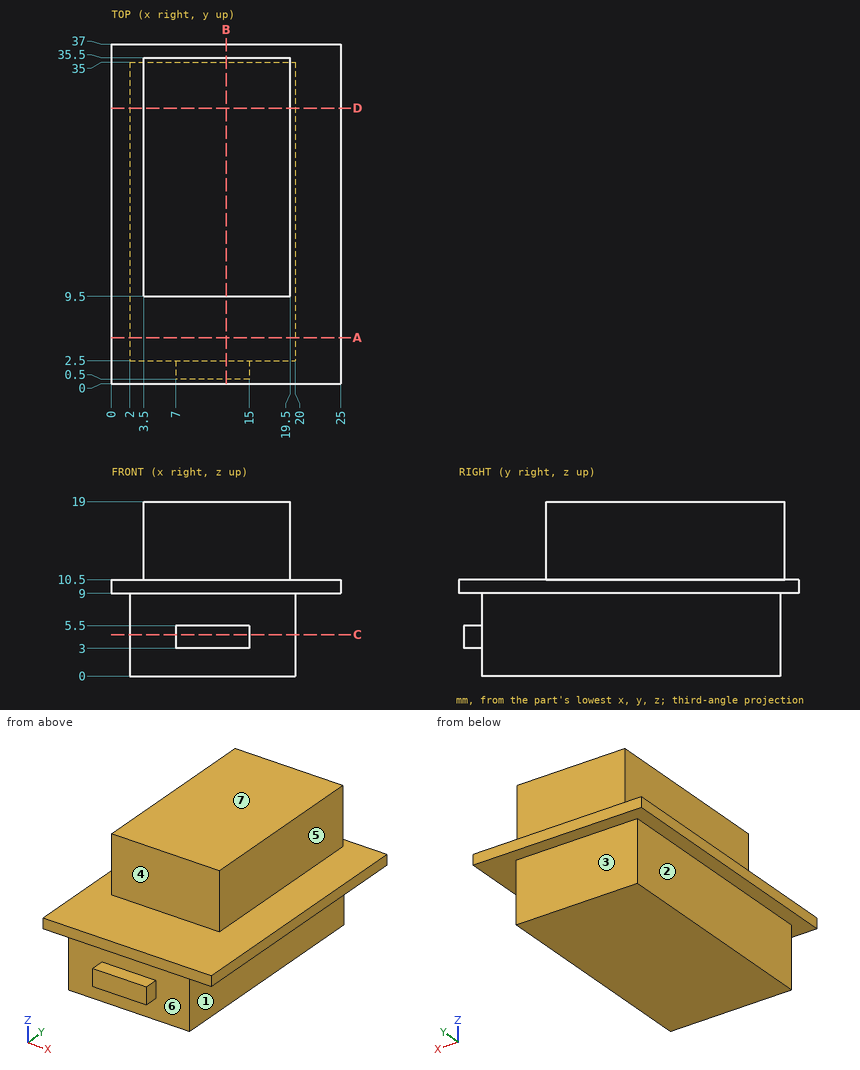
Answer from the drawing. Dimensions are ordinates in mm from the lowest x, y and z of the part. A direction names the side the tool comes from. Coordinates: 2 decimals unless noted, no trailing zeros. Loops run counter-clockwise (first coordinate to the right, second up) from the corner with the lowest first, then second, coordinate; pieces in that order, holes last. Notation, with made-up numbers: (22.5, 78) -> (38.5, 78) arc R20 cw to (38.5, 116) -> close; hole circle Ø8 at (25, -5). An arc over 180 degrees is marked (long way). Answer as CSV lines item,"result".
Q1. The part is cut by section C-C on z = 4.5. Write down the section's boundary in (x, y).
Findings:
outline,"(2, 2.5) -> (7, 2.5) -> (7, 0.5) -> (15, 0.5) -> (15, 2.5) -> (20, 2.5) -> (20, 35) -> (2, 35) -> close"
Q2. The part is cut by section D-D on y = 30. Write down the section's boundary in (x, z).
Findings:
outline,"(0, 9) -> (2, 9) -> (2, 0) -> (20, 0) -> (20, 9) -> (25, 9) -> (25, 10.5) -> (19.5, 10.5) -> (19.5, 19) -> (3.5, 19) -> (3.5, 10.5) -> (0, 10.5) -> close"
Q3. The part is cut by section B-B on x = 12.5. Write down the section's boundary in (y, z).
Findings:
outline,"(0, 9) -> (2.5, 9) -> (2.5, 5.5) -> (0.5, 5.5) -> (0.5, 3) -> (2.5, 3) -> (2.5, 0) -> (35, 0) -> (35, 9) -> (37, 9) -> (37, 10.5) -> (35.5, 10.5) -> (35.5, 19) -> (9.5, 19) -> (9.5, 10.5) -> (0, 10.5) -> close"
Q4. For a pull along Z with two mould halves and no side action, classify the marked faces 5, 6 and 7 as +Z half, -Z half, draft (parallel to the pull), parting line (faces both ways), or undercut.
Findings:
face 5,"draft"
face 6,"undercut"
face 7,"+Z half"
Q5. The part is cut by section A-A on y = 5. Write down the section's boundary in (x, z), and give its area (4 significant figures).
Findings:
outline,"(0, 9) -> (2, 9) -> (2, 0) -> (20, 0) -> (20, 9) -> (25, 9) -> (25, 10.5) -> (0, 10.5) -> close"
area,"199.5 mm²"
Q6. Find the intervals of material crossed by probe 1 along Y at (x, z) = (11, 2.5); probe 2 along Z at (x, y) = (3.25, 24); probe 3 along X at (y, z) = (28.5, 12), in increasing order.
Findings:
probe 1,"y = 2.5 to 35"
probe 2,"z = 0 to 10.5"
probe 3,"x = 3.5 to 19.5"
Q7. Each of these flat-tipped pins is pushed along its axis until it touches: pin 1 (2.5 mm diameter, centred on y = 18.5, z = 15.5, fed in from -X); pin 2 (2 mm diameter, centred on x = 13.5, z = 5.5, fed in from -Y); pin 3 (1 mm diameter, centred on x = 12, z = 8, fed in from -Y). Where does it stop, or does it pass through?
Findings:
pin 1,"stops at x = 3.5"
pin 2,"stops at y = 0.5"
pin 3,"stops at y = 2.5"
Q8. A tool of negligible diameter and unlimited length cuts with its end or side. For the marked faces 1, 2, 3 and 4, from which of +Z, -Z, +X, -X, +Y, -Y can it reach the whole face along a straight path? Write none if from no direction.
Findings:
face 1,"-Z, +X, +Y, -Y"
face 2,"-Z, -X, +Y, -Y"
face 3,"-Z, +X, -X, +Y"
face 4,"+Z, +X, -X, -Y"
